Job drawing, mm, ordinate dimensions from the low corner. One solid piece. Coordinates: 2 decimals unless noted, no trailing zeros. Write each loop counter-clockwise with the first axis right and the second up, starting at its lowest first coordinate (ties: lowest second). Pieces come first, ordered by that corner, then holes. Notation, with made-up numbers: (-1, 24) - (9, 24) arc R27 ccw to (9, 59) - close; hole circle Ø9 at (39.25, 43). An arc over 180 degrees is marked (long way). Use a Markdown table: item, result.
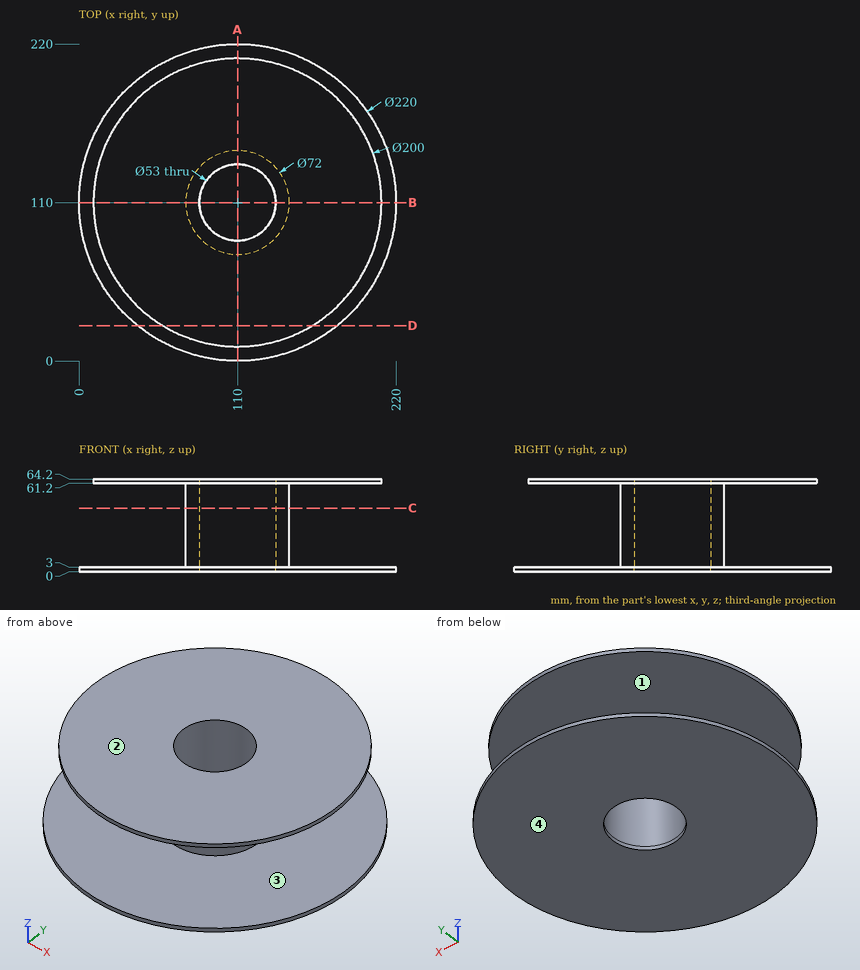
Item 1: Band-saw the part on D-D, the plane y = 24.5. Give the cut face in (x, z).
From the geometry:
| item | result |
|---|---|
| outline | (40.79, 0) - (179.21, 0) - (179.21, 3) - (40.79, 3) - close; (58.14, 61.2) - (161.86, 61.2) - (161.86, 64.2) - (58.14, 64.2) - close |
Item 2: Drill centre lines: probe 1 along Z at (x, y) = (169.5, 117); probe 2 along Y at (x, z) = (110, 2.45); probe 3 along Y at (x, z) = (110, 25). Where is each one in solid material? Low to high.
From the geometry:
| item | result |
|---|---|
| probe 1 | 0 to 3, 61.2 to 64.2 |
| probe 2 | 0 to 83.5, 136.5 to 220 |
| probe 3 | 74 to 83.5, 136.5 to 146 |
Item 3: Two-plate mould, pull along Z, no slides. Class the marked faces 1, 2, 3 and 4: pulls with the +Z half, pulls with the -Z half, needs draft (parallel to the pull), parting line crosses it, or undercut.
From the geometry:
| item | result |
|---|---|
| face 1 | undercut |
| face 2 | pulls with the +Z half |
| face 3 | undercut |
| face 4 | pulls with the -Z half |
Item 4: Drop flat-ended pins along their axis: P1, Ø2, axis at y = 117.5, z = 27, coming from the -X side; P2, Ø8, axis at x = 61.5, y = 168, coming from the -Z side; P3, Ø6, axis at x = 142, z = 28, coming from the -Y side. Give the stop position or say it passes through.
From the geometry:
| item | result |
|---|---|
| P1 | x = 74.59 |
| P2 | z = 0 |
| P3 | y = 88.67 |
Item 5: Band-saw the part on A-A, the plane x = 110. Give the cut face in (y, z).
From the geometry:
| item | result |
|---|---|
| outline | (0, 0) - (83.5, 0) - (83.5, 64.2) - (10, 64.2) - (10, 61.2) - (74, 61.2) - (74, 3) - (0, 3) - close; (136.5, 0) - (220, 0) - (220, 3) - (146, 3) - (146, 61.2) - (210, 61.2) - (210, 64.2) - (136.5, 64.2) - close |
Item 6: Band-saw the part on C-C, the plane z = 44. Give the cut face in (x, y).
From the geometry:
| item | result |
|---|---|
| outline | circle Ø72 at (110, 110); hole circle Ø53 at (110, 110) |
